The model under review builds one solid part; all positions refer to its coordinate system, in mm. Coordinates: 2 decimals unless noted, no trailing zeros. Loops run counter-clockwise (first coordinate to the right, second up) from the corner with the lowest first, then second, coordinate; pieces in that order, holes last. Notation, with made-up numbers: (82, 69) - (100, 69) arc R18 cw to (100, 97) - close; hole circle Ø5 at (57, 12.5). An arc over 180 degrees is marked (long way). One line per item, written item: value. Start each with the question number.
1. To check wall thickness, follow line 1 (Y direction, x = -3, z = -6.35) (3 decimals); line 2 (Y direction, x = -1, z = -6.35) (3 decimals); line 3 (Y direction, x = -3.8, z = -6). State the ranges of each line that lie inside material, in increasing order.
2. We need section C-C, the plane y = 6. Give the boundary of the cut face in (x, z).
3. Mouldability with a two-part tool opening along Z and no side actions: class faces 1 (the face through (-1.97, 7.16, -6.15)), 2 (the face through (-3, 0, -12.7)), 3 (the face through (-2, 8.85, -6)), 4 (the face through (-3, 0, 0)) as +Z half, -Z half, draft (parallel to the pull), parting line (faces both ways), or undercut.
4. We need section B-B, the plane z = -6.35. Give the boundary of the cut face in (x, y) (3 decimals).
5. We need section D-D, the plane z = -8.25. Give the boundary of the cut face in (x, y).
6. We need section A-A, the plane x = -1.1. Give the boundary of the cut face in (y, z) (3 decimals).
from build123d import *

# Parameters (mm, degrees)
SKETCH1_W           = 4
SKETCH1_H           = 12.7
BOSS_EXTRUDE1_DEPTH = 8.85
SKETCH2_R           = 2.5
CUT_EXTRUDE1_DEPTH  = 16.987886039
SKETCH3_R           = 1.5
CUT_EXTRUDE2_DEPTH  = 16.987886039


with BuildPart() as part:
    # Sketch1 → Boss-Extrude1 (new, symmetric)
    with BuildSketch(Plane(origin=(0, 0, 0), x_dir=(1, 0, 0), z_dir=(0, 1, 0))):
        with Locations((-2, 6.35)):
            Rectangle(SKETCH1_W, SKETCH1_H)
    extrude(amount=BOSS_EXTRUDE1_DEPTH, both=True)

    # Sketch2 → Cut-Extrude1 (cut, through all)
    with BuildSketch(Plane.XY):
        Circle(SKETCH2_R)
    extrude(amount=-CUT_EXTRUDE1_DEPTH, mode=Mode.SUBTRACT)

    # Sketch3 → Cut-Extrude2 (cut, through all)
    with BuildSketch(Plane(origin=(0, 0, 0), x_dir=(0, 0, -1), z_dir=(1, 0, 0))):
        with Locations((6.35, 5.675)):
            Circle(SKETCH3_R)
        with Locations((6.35, -5.675)):
            Circle(SKETCH3_R)
    extrude(amount=-CUT_EXTRUDE2_DEPTH, mode=Mode.SUBTRACT)


solid = part.part
Findings below:
1. line 1: -8.85 to -7.175, -4.175 to 4.175, 7.175 to 8.85
1. line 2: -8.85 to -7.175, -4.175 to -2.291, 2.291 to 4.175, 7.175 to 8.85
1. line 3: -8.85 to -7.13, -4.22 to 4.22, 7.13 to 8.85
2. outline: (-4, -12.7) - (0, -12.7) - (0, -7.81) - (-4, -7.81) - close; (-4, -4.89) - (0, -4.89) - (0, 0) - (-4, 0) - close
3. face 1: undercut
3. face 2: -Z half
3. face 3: draft
3. face 4: +Z half
4. outline: (-4, -8.85) - (0, -8.85) - (0, -7.175) - (-4, -7.175) - close; (-4, -4.175) - (0, -4.175) - (0, -2.5) arc R2.5 cw to (0, 2.5) - (0, 4.175) - (-4, 4.175) - close; (-4, 7.175) - (0, 7.175) - (0, 8.85) - (-4, 8.85) - close
5. outline: (-4, -8.85) - (0, -8.85) - (0, -2.5) arc R2.5 cw to (0, 2.5) - (0, 8.85) - (-4, 8.85) - close
6. outline: (-8.85, -12.7) - (-2.245, -12.7) - (-2.245, 0) - (-8.85, 0) - close; (2.245, -12.7) - (8.85, -12.7) - (8.85, 0) - (2.245, 0) - close; hole circle Ø3 at (-5.675, -6.35); hole circle Ø3 at (5.675, -6.35)
